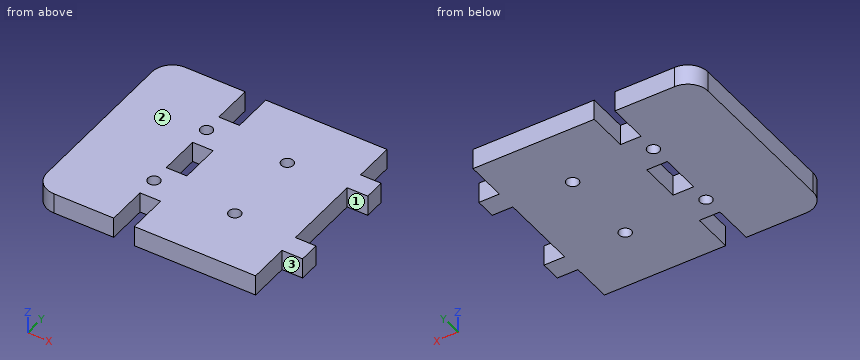
Autodesk Inventor part; units mm, degrees
ref_plane "YZ Plane" through (0, 0, 0) normal (1, 0, 0) x (0, 1, 0)
ref_plane "XZ Plane" through (0, 0, 0) normal (0, 1, 0) x (-1, 0, 0)
ref_plane "XY Plane" through (0, 0, 0) normal (0, 0, 1) x (1, 0, 0)
sketch "Sketch1" plane through (0, 0, 0) normal (0, 0, 1) x (1, 0, 0)
  line L0 (30, -25) -> (-25, -25)
  line L1 (-30, -20) -> (-30, 20)
  line L2 (-25, 25) -> (30, 25)
  line L3 (30, 25) -> (30, -25)
  line L4 (30, -25) -> (-30, 25) construction
  line L5 (-30, -25) -> (30, 25) construction
  circle A0 centre (-10, 10) radius 1.5
  circle A1 centre (-10, -10) radius 1.5
  circle A2 centre (10, 10) radius 1.5
  circle A3 centre (10, -10) radius 1.5
  arc A4 (-25, 25) -> (-30, 20) centre (-25, 20) ccw
  arc A5 (-30, -20) -> (-25, -25) centre (-25, -20) ccw
  point P0 (0, 0)
  dimension "d0" = 60
  dimension "d1" = 50
  dimension "d2" = 3
  dimension "d3" = 3
  dimension "d4" = 3
  dimension "d5" = 3
  dimension "d6" = 10
  dimension "d7" = 10
  dimension "d8" = 10
  dimension "d9" = 10
  dimension "d10" = 10
  dimension "d11" = 10
  dimension "d12" = 10
  dimension "d13" = 10
  dimension "d14" = 5
extrude "Extrusion1" add sketch "Sketch1" along normal blind 5.1
sketch "Sketch4" plane through (0, 0, 0) normal (0, 0, -1) x (-1, 0, 0)
  line L0 (-30, 25) -> (25, 25)
  line L1 (-30, 25) -> (-24.9, 25)
  line L2 (-24.9, 25) -> (-24.9, 14.95)
  line L3 (-24.9, 14.95) -> (-30, 14.95)
  line L4 (-30, 14.95) -> (-30, 25)
  line L5 (-30, -25) -> (-30, 25)
  line L6 (-30, 9.85) -> (-24.9, 9.85)
  line L7 (-24.9, 9.85) -> (-24.9, -9.85)
  line L8 (-24.9, -9.85) -> (-30, -9.85)
  line L9 (-30, -9.85) -> (-30, 9.85)
  line L10 (25, -25) -> (-30, -25)
  line L11 (-30, -25) -> (-24.9, -25)
  line L12 (-24.9, -25) -> (-24.9, -14.95)
  line L13 (-24.9, -14.95) -> (-30, -14.95)
  line L14 (-30, -14.95) -> (-30, -25)
  point P0 (0, 0)
  point P1 (-24.9, 0)
  point P2 (-30, 0)
  dimension "d27" = 5.1
  dimension "d28" = 10.05
  dimension "d29" = 5.1
  dimension "d30" = 19.7
  dimension "d31" = 10.05
  dimension "d32" = 5.1
extrude "Extrusion5" cut sketch "Sketch4" against normal blind 40
sketch "Sketch5" plane through (0, 0, 5.1) normal (0, 0, 1) x (1, 0, 0)
  circle A0 centre (10, -10) radius 1.5
  circle A1 centre (10, 10) radius 1.5
  line L0 (24.9, -25) -> (24.9, -14.95)
  line L1 (24.9, -14.95) -> (30, -14.95)
  line L2 (30, -14.95) -> (30, -9.85)
  line L3 (30, -9.85) -> (24.9, -9.85)
  line L4 (24.9, -9.85) -> (24.9, 9.85)
  line L5 (24.9, 9.85) -> (30, 9.85)
  line L6 (30, 9.85) -> (30, 14.95)
  line L7 (30, 14.95) -> (24.9, 14.95)
  line L8 (24.9, 14.95) -> (24.9, 25)
  line L9 (24.9, 25) -> (-25, 25)
  arc A2 (-25, 25) -> (-30, 20) centre (-25, 20) ccw
  line L10 (-30, 20) -> (-30, -20)
  arc A3 (-30, -20) -> (-25, -25) centre (-25, -20) ccw
  line L11 (-25, -25) -> (24.9, -25)
  line L12 (-10.2, 5) -> (-5.1, 5)
  line L13 (-5.1, 5) -> (-5.1, -5)
  line L14 (-5.1, -5) -> (-10.2, -5)
  line L15 (-10.2, -5) -> (-10.2, 5)
  line L16 (-10.2, -15) -> (-5.1, -15)
  line L17 (-5.1, -15) -> (-5.1, -25)
  line L18 (-5.1, -25) -> (-10.2, -25)
  line L19 (-10.2, -25) -> (-10.2, -15)
  line L20 (-10.2, 15) -> (-5.1, 15)
  line L21 (-5.1, 15) -> (-5.1, 25)
  line L22 (-5.1, 25) -> (-10.2, 25)
  line L23 (-10.2, 25) -> (-10.2, 15)
  line L24 (-43.2426, 0) -> (42.2071, 0) construction
  point P0 (0, 0)
  dimension "d35" = 5.1
  dimension "d36" = 5.1
  dimension "d37" = 5.1
  dimension "d38" = 19.7
  dimension "d40" = 30
  dimension "d43" = 10
  dimension "d44" = 10
extrude "Extrusion6" cut sketch "Sketch5" against normal through all contours L11 L19 L16 L17 | L9 L21 L20 L23 | L12 L13 L14 L15
equation "\"d36\" = d35"
equation "\"d37\" = d36"
equation "\"d44\" = d43"
properties part number "motor chasis holder" material "Polycarbonate, Smoke"
Source: CAD feature listing. Evaluate the final solid. Frame: model axes, mm. Face numbers are marked on the shaded views. Round coordinates to 2 decimals unless told otherwise and drop trailing zeros. Loops run counter-clockwise (first coordinate to the right, second up) from the corner with the lowest first, then second, coordinate; pieces in that order, holes last. Notation, with made-up numbers: M 76.5,34 L 133.5,34 A24 cw 133.5,71 Z; hole C -35.75,-9 d2. An arc over 180 degrees is marked long. Use a Markdown table: item, result. Add a question column.
1. Cut plane C-C, the plane y = -2. Output: boundary loops of the cut face in (x, z), and give its area (3 significant figures).
2. Cut plane D-D, the plane x = 10. Output: boundary loops of the cut face in (y, z).
3. Contact query for flat-ended pins moving along their axis: pin 1 (2.5 mm diameter, centred on x = 28, z = 2.5, fed in from +Y); pin 2 (1.5 mm diameter, centred on x = -8.5, z = 2.5, fed in from +Y); pin 3 (1.5 mm diameter, centred on y = 0.5, z = 1.5, fed in from +X). Output: stop coordinate, or through.
4. Cut plane A-A, the plane x = -6.5. Output: boundary loops of the cut face in (y, z).
5. Cut plane B-B, the plane z = 3.6. State how many separate pieces and enclosed holes the cut face has, and give its area (3 significant figures).
6. Ray query, line 1 along Y through (x, z) = (10, 2.35); line 2 along Y through (x, z) = (-10, 2.55); line 3 along X through (y, z) = (-19.5, 3.65). Return the intervals inside material, ascending. Write a range as [from, to].
7. Pull-direction query (Y, two-part tool) for the marked faces 1, 2 and 3; classes: +Y half, -Y half, draft (parallel to the pull), parting line (faces both ways), or undercut.
Solution:
| question | item | result |
|---|---|---|
| 1 | outline | M -30,0 L -10.2,0 L -10.2,5.1 L -30,5.1 Z; M -5.1,0 L 24.9,0 L 24.9,5.1 L -5.1,5.1 Z |
| 1 | area | 254 mm2 |
| 2 | outline | M -25,0 L -11.5,0 L -11.5,5.1 L -25,5.1 Z; M -8.5,0 L 8.5,0 L 8.5,5.1 L -8.5,5.1 Z; M 11.5,0 L 25,0 L 25,5.1 L 11.5,5.1 Z |
| 3 | pin 1 | stops at y = 14.95 |
| 3 | pin 2 | stops at y = 15 |
| 3 | pin 3 | stops at x = 24.9 |
| 4 | outline | M -15,0 L -5,0 L -5,5.1 L -15,5.1 Z; M 5,0 L 15,0 L 15,5.1 L 5,5.1 Z |
| 5 | separate pieces | 1 |
| 5 | enclosed holes | 5 |
| 5 | area | 2,610 mm2 |
| 6 | line 1 | y = [-25, -11.5], [-8.5, 8.5], [11.5, 25] |
| 6 | line 2 | y = [-15, -11.5], [-8.5, -5], [5, 8.5], [11.5, 15] |
| 6 | line 3 | x = [-30, -10.2], [-5.1, 24.9] |
| 7 | face 1 | undercut |
| 7 | face 2 | draft |
| 7 | face 3 | -Y half |
